```python
from build123d import *

# Parameters (mm, degrees)
SKETCH_1_W          = 30
SKETCH_1_H          = 30
EXTRUDE_1_DEPTH     = 15
SKETCH_2_R          = 4
CUT_EXTRUDE_1_DEPTH = 46
SKETCH_3_W          = 10
SKETCH_3_H          = 15
CUT_EXTRUDE_2_DEPTH = 46


with BuildPart() as part:
    # 草图1 → 凸台-拉伸1 (new body)
    with BuildSketch(Plane.XY):
        with Locations((15, 15)):
            Rectangle(SKETCH_1_W, SKETCH_1_H)
    extrude(amount=EXTRUDE_1_DEPTH)

    # 草图2 → 切除-拉伸1 (cut, through all)
    with BuildSketch(Plane.XY.offset(15)):
        with Locations((7, 7)):
            Circle(SKETCH_2_R)
    extrude(amount=-CUT_EXTRUDE_1_DEPTH, mode=Mode.SUBTRACT)

    # 草图3 → 切除-拉伸2 (cut, through all)
    with BuildSketch(Plane.ZY):
        with Locations((10, 7.5)):
            Rectangle(SKETCH_3_W, SKETCH_3_H)
    extrude(amount=-CUT_EXTRUDE_2_DEPTH, mode=Mode.SUBTRACT)


solid = part.part
```
Check sheet for the modelled part. Datum: model origin and axes. Units: mm. A direction names the side the tool comes from. Coordinates: 2 decimals unless noted, no trailing zeros. Order: outer loops, then holes, each group sorted by start corner. A loop starts at its lowest first (then second) coordinate and runs counter-clockwise, first axis right, second up. Notation, with made-up numbers: M 14,7 L 67,7 A23 ccw 67,31 Z; hole C -1,59 d6. An arc over 180 degrees is marked long. One line per question, with ' | ' between items. Start each with the question number.
Item 1: Access from +Z, -Z, +X, -X, +Y, -Y to the whole of each face (thin tool, end or side, straight path). Record for faces 1 (the flat face through (15, 15, 0)), 2 (the flat face through (15, 15, 10)).
Item 2: Sectioned sample at B-B on y = 7. Record the cut outline in (x, z), and give its area (3 significant figures).
Item 3: Sectioned sample at A-A on x = 7. Record the cut outline in (y, z).
Item 4: Sectioned sample at C-C on z = 3. Record the cut outline in (x, y), and give its area (3 significant figures).
Item 5: Gauge pin test, flat ends, axial feed: P1, Ø8, axis at x = 9.5, y = 7.5, coming from the +Z side; P2, Ø5, axis at x = 17, z = 12, coming from the -Y side. Record the tip position at first contact, or that the pin passes through.
Item 6: Material ranges on line 1 (Y direction, x = 7, z = 2); line 2 (Y direction, x = 26.25, z = 5.5); line 3 (Z direction, x = 22.75, y = 1.5), recorded low to high.
Item 7: Sectioned sample at D-D on x = 27.25. Record the cut outline in (y, z), and give its area (3 significant figures).
Answer below:
1) face 1: -Z, +X, -X, +Y, -Y | face 2: +Z, +X, -X, -Y
2) outline: M 0,0 L 3,0 L 3,5 L 0,5 Z; M 11,0 L 30,0 L 30,5 L 11,5 Z | area: 110 mm^2
3) outline: M 0,0 L 3,0 L 3,5 L 0,5 Z; M 11,0 L 30,0 L 30,15 L 15,15 L 15,5 L 11,5 Z
4) outline: M 0,0 L 30,0 L 30,30 L 0,30 Z; hole C 7,7 d8 | area: 850 mm^2
5) P1: stops at z = 5 | P2: stops at y = 15
6) line 1: y = 0 to 3, 11 to 30 | line 2: y = 15 to 30 | line 3: z = 0 to 5
7) outline: M 0,0 L 30,0 L 30,15 L 15,15 L 15,5 L 0,5 Z | area: 300 mm^2
